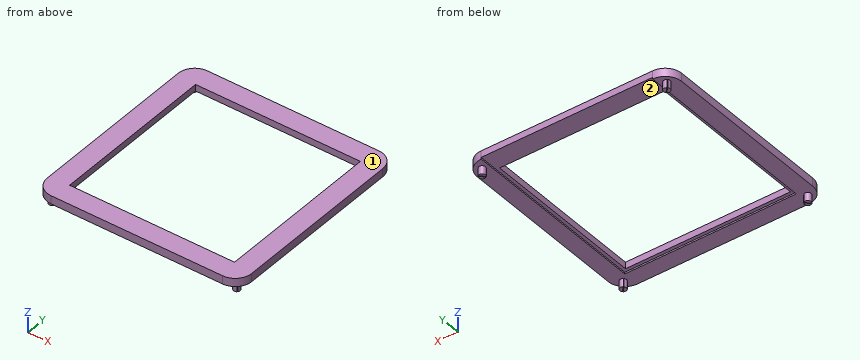
```python
from build123d import *

# Parameters (mm, degrees)
F0_R          = 1
F0_W          = 52
F0_H          = 52
F0_W_2        = 50
F0_H_2        = 50
F1_DEPTH      = 2.5
F2_DEPTH      = 0.5
F3_W          = 52
F3_H          = 5
F4_DEPTH      = 0.5
F5_DEPTH      = 2.5
F5_DEPTH_BACK = 2.5
F7_DEPTH      = 2.5
F9_DEPTH      = 2.5


with BuildPart() as f1:
    # F0 (on Top) → F1 (new body)
    with BuildSketch(Plane.XY):
        with BuildLine():
            Line((57, 0), (5, 0))
            ThreePointArc((5, 0), (1.4644660941, -1.4644660941), (0, -5))
            Line((0, -5), (0, -57))
            ThreePointArc((0, -57), (1.4644660941, -60.5355339059), (5, -62))
            Line((5, -62), (57, -62))
            ThreePointArc((57, -62), (60.5355339059, -60.5355339059), (62, -57))
            Line((62, -57), (62, -5))
            ThreePointArc((62, -5), (60.5355339059, -1.4644660941), (57, 0))
        make_face()
        with Locations((3, -59)):
            Circle(F0_R, mode=Mode.SUBTRACT)
        with Locations((59, -59)):
            Circle(F0_R, mode=Mode.SUBTRACT)
        with Locations((3, -3)):
            Circle(F0_R, mode=Mode.SUBTRACT)
        with Locations((31, -31)):
            Rectangle(F0_W, F0_H, mode=Mode.SUBTRACT)
        with Locations((59, -3)):
            Circle(F0_R, mode=Mode.SUBTRACT)
        with Locations((31, -31)):
            Rectangle(F0_W, F0_H)
        with Locations((31, -31)):
            Rectangle(F0_W_2, F0_H_2, mode=Mode.SUBTRACT)
    extrude(amount=F1_DEPTH)

    # F0 (on Top) → F2 (cut)
    with BuildSketch(Plane.XY):
        with Locations((31, -31)):
            Rectangle(F0_W, F0_H)
        with Locations((31, -31)):
            Rectangle(F0_W_2, F0_H_2, mode=Mode.SUBTRACT)
    extrude(amount=F2_DEPTH, mode=Mode.SUBTRACT)

    # F3 (on face) → F4 (cut)
    with BuildSketch(Plane.XY):
        with Locations((31, -2.5)):
            Rectangle(F3_W, F3_H)
    extrude(amount=F4_DEPTH, mode=Mode.SUBTRACT)

    # F0 (on Top) → F5 (join, two sides)
    with BuildSketch(Plane.XY) as f5_sk:
        with Locations((59, -59)):
            Circle(F0_R)
        with Locations((59, -3)):
            Circle(F0_R)
        with Locations((3, -3)):
            Circle(F0_R)
        with Locations((3, -59)):
            Circle(F0_R)
    extrude(amount=F5_DEPTH)
    extrude(f5_sk.sketch, amount=-F5_DEPTH_BACK)

    # F6 (on face) → F7 (cut)
    with BuildSketch(Plane(origin=(0, 0, -2.5), x_dir=(1, 0, 0), z_dir=(0, 0, -1))):
        with BuildLine():
            ThreePointArc((58.3671483141, 3.7742730421), (58.2928932188, 3.7071067812), (58.2257269579, 3.6328516859))
            Line((58.2257269579, 3.6328516859), (59.6328516859, 2.2257269579))
            ThreePointArc((59.6328516859, 2.2257269579), (59.7071067812, 2.2928932188), (59.7742730421, 2.3671483141))
            Line((59.7742730421, 2.3671483141), (58.3671483141, 3.7742730421))
        make_face()
    extrude(amount=-F7_DEPTH, mode=Mode.SUBTRACT)

    # F8 (on face) → F9 (cut)
    with BuildSketch(Plane(origin=(0, 0, -2.5), x_dir=(1, 0, 0), z_dir=(0, 0, -1))):
        with BuildLine():
            ThreePointArc((58.2221825407, 58.3636038969), (58.2221825407, 58.2221825407), (58.3636038969, 58.2221825407))
            Line((58.3636038969, 58.2221825407), (59.7778174593, 59.6363961031))
            ThreePointArc((59.7778174593, 59.6363961031), (59.7778174593, 59.7778174593), (59.6363961031, 59.7778174593))
            Line((59.6363961031, 59.7778174593), (58.2221825407, 58.3636038969))
        make_face()
        with BuildLine():
            ThreePointArc((2.2221825407, 2.3636038969), (2.2221825407, 2.2221825407), (2.3636038969, 2.2221825407))
            Line((2.3636038969, 2.2221825407), (3.7778174593, 3.6363961031))
            ThreePointArc((3.7778174593, 3.6363961031), (3.7778174593, 3.7778174593), (3.6363961031, 3.7778174593))
            Line((3.6363961031, 3.7778174593), (2.2221825407, 2.3636038969))
        make_face()
        with BuildLine():
            ThreePointArc((2.3671483141, 59.7742730421), (2.2928932188, 59.7071067812), (2.2257269579, 59.6328516859))
            Line((2.2257269579, 59.6328516859), (3.6328516859, 58.2257269579))
            ThreePointArc((3.6328516859, 58.2257269579), (3.7071067812, 58.2928932188), (3.7742730421, 58.3671483141))
            Line((3.7742730421, 58.3671483141), (2.3671483141, 59.7742730421))
        make_face()
    extrude(amount=-F9_DEPTH, mode=Mode.SUBTRACT)


solid = f1.part
```
Read the model definition and answer for the solid it produces. Units are mm, in the model's axes. Face numbers are marked on the shaded views. Round coordinates to 2 decimals unless told otherwise and drop trailing zeros. Write each loop counter-clockwise with the first axis right and the second up, starting at its lowest first coordinate (ties: lowest second). Pieces come first, ordered by that corner, then holes. Notation, with made-up numbers: M 56.5,35 L 81.5,35 A9 ccw 81.5,42 Z; hole C 83.5,58 d11. An arc over 180 degrees is marked long. One line per item, written item: value.
Q1. Straight lines are drawn through the part: line 1 (Y direction, x = 33.5, z = 0.65); line 2 (X direction, y = -7, z = 0.9); line 3 (X direction, y = -6, z = 0.15). For each, find the intervals that lie inside material, in ascending order. Write a range as [from, to].
Data:
line 1: [-62, -56], [-6, 0]
line 2: [0, 6], [56, 62]
line 3: [0, 5], [57, 62]
Q2. A flat-ended cylindrical pin translates along its axis: pin 1 Ø2 at (x, z) = (14.5, -1.5) entering from -Y. Find the tip coordinate at first contact, or state that the pin passes through.
Data:
pin 1: through
Q3. For a pull along X with two mould halves and no side action, classify the marked faces 1 and 2 as +X half, -X half, draft (parallel to the pull), parting line (faces both ways), or undercut.
Data:
face 1: draft
face 2: undercut
Q4. Find section A-A on x = 31.5. Write down the section's boundary in (y, z).
Data:
outline: M -62,0 L -57,0 L -57,0.5 L -56,0.5 L -56,2.5 L -62,2.5 Z; M -6,0.5 L 0,0.5 L 0,2.5 L -6,2.5 Z
Q5. Find section C-C on y = -35. Write down the section's boundary in (x, z), plus the area to 3 significant figures.
Data:
outline: M 0,0 L 5,0 L 5,0.5 L 6,0.5 L 6,2.5 L 0,2.5 Z; M 56,0.5 L 57,0.5 L 57,0 L 62,0 L 62,2.5 L 56,2.5 Z
area: 29.0 mm2
